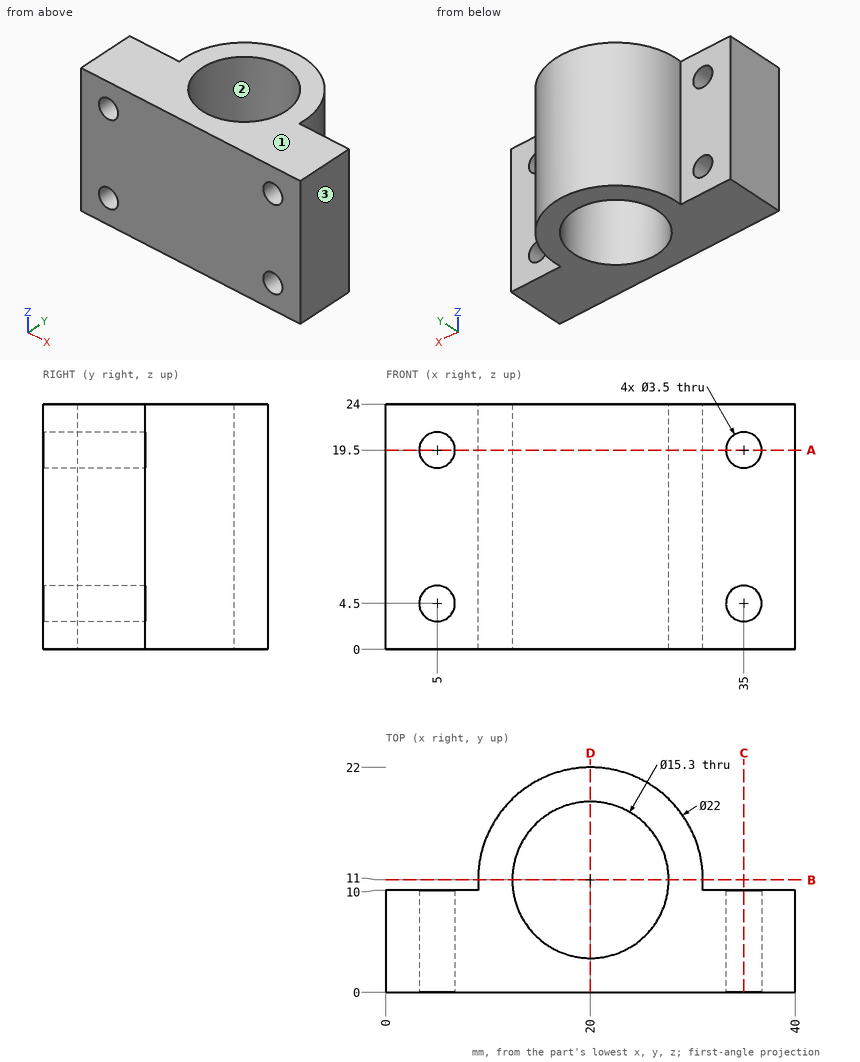
Verification items for this drawing (mm, ordinates from the low corner). Give positions to 0.01 mm unless a question says otherwise; leave off trailing zeros. Write each loop counter-clockwise with the first axis right and the second up, starting at its lowest first coordinate (ties: lowest second). Pieces come first, ordered by that corner, then holes. Notation, with made-up numbers: (53.5, 36.25) -> (79.5, 36.25) arc R14 cw to (79.5, 47.25) -> close; hole circle Ø2 at (53.25, -38.5). An arc over 180 degrees is marked (long way). Use CSV: the item, a comma, the result in double quotes. Start each with the question number.
Q1. Depth check by flat-ended pin: P1, Ø5, axis at y = 16, z = 16.5, coming from the -X side; P2, Ø6, axis at x = 10, z = 20.5, coming from the +Y side; P3, Ø2, axis at x = 35, z = 19.5, coming from the +Y side; P4, Ø10, axis at x = 6.5, z = 15, coming from the +Y side. Enter the tip coordinate at first touch or a pass-through.
Q2. Cross-section at B-B on y = 11. Enter the section's corners in (x, z).
Q3. Scan lines: line 1 along X through (y, z) = (4.75, 4.5); line 2 along X through (y, z) = (6.25, 19.5); line 3 along Y through (x, z) = (4, 15.5). Record each from-to range of solid material in increasing order.
Q4. Cross-section at D-D on x = 20. Enter the section's corners in (y, z), and give its area (3 significant figures).
Q5. Cross-section at C-C on x = 35. Enter the section's corners in (y, z).
Q6. Cross-section at A-A on z = 19.5. Enter the section's corners in (x, y), and give its area (3 significant figures).
Q7. Release check for a two-part mould opening along X. For the marked faces 1, 2 and 3 record: +X half, -X half, draft (parallel to the pull), parting line (faces both ways), or undercut.
Working result:
1,P1,"stops at x = 9.29"
1,P2,"stops at y = 19.49"
1,P3,"passes through"
1,P4,"stops at y = 17.98"
2,outline,"(9, 0) -> (12.35, 0) -> (12.35, 24) -> (9, 24) -> close; (27.65, 0) -> (31, 0) -> (31, 24) -> (27.65, 24) -> close"
3,line 1,"x = 0 to 3.25, 6.75 to 15.59, 24.41 to 33.25, 36.75 to 40"
3,line 2,"x = 0 to 3.25, 6.75 to 14, 26 to 33.25, 36.75 to 40"
3,line 3,"y = 0 to 10"
4,outline,"(0, 0) -> (3.35, 0) -> (3.35, 24) -> (0, 24) -> close; (18.65, 0) -> (22, 0) -> (22, 24) -> (18.65, 24) -> close"
4,area,"161 mm^2"
5,outline,"(0, 0) -> (10, 0) -> (10, 2.75) -> (0, 2.75) -> close; (0, 6.25) -> (10, 6.25) -> (10, 17.75) -> (0, 17.75) -> close; (0, 21.25) -> (10, 21.25) -> (10, 24) -> (0, 24) -> close"
6,outline,"(0, 0) -> (3.25, 0) -> (3.25, 10) -> (0, 10) -> close; (6.75, 0) -> (33.25, 0) -> (33.25, 10) -> (30.95, 10) arc R11 ccw (long way) to (9.05, 10) -> (6.75, 10) -> close; (36.75, 0) -> (40, 0) -> (40, 10) -> (36.75, 10) -> close; hole circle Ø15.3 at (20, 11)"
6,area,"358 mm^2"
7,face 1,"draft"
7,face 2,"undercut"
7,face 3,"+X half"
